```python
from build123d import *

# Parameters (mm, degrees)
EXTRUDE_1_DEPTH      = 1.5
CUT_EXTRUDE_1_DEPTH  = 1.5
SKETCH_3_R           = 2
CUT_EXTRUDE_2_DEPTH  = 1.5
SKETCH_4_W           = 80
SKETCH_4_H           = 5
EXTRUDE_2_DEPTH      = 1.5
FILLET_1_R           = 2
SKETCH_5_OUTSIDE_W   = 163.618
SKETCH_5_OUTSIDE_H   = 213.618
SKETCH_5_OUTSIDE_W_2 = 80
SKETCH_5_OUTSIDE_H_2 = 170
CUT_EXTRUDE_3_DEPTH  = 193.943644622
SKETCH_6_R           = 1.5
CUT_EXTRUDE_4_DEPTH  = 184.377343202


with BuildPart() as part:
    # 草图1 → 凸台-拉伸1 (new body)
    with BuildSketch(Plane.XY):
        Polygon((80, 90), (100, 90), (100, 70), (80, 70), (80, 0), (0, 0), (0, 70), (-20, 70), (-20, 90), (0, 90), (0, 160), (80, 160), align=None)
    extrude(amount=EXTRUDE_1_DEPTH)

    # 草图2 → 切除-拉伸1 (cut)
    with BuildSketch(Plane.XY.offset(1.5)):
        with BuildLine():
            Line((57.5, 152.25), (80, 152.25))
            Line((80, 152.25), (80, 157.75))
            Line((80, 157.75), (57.5, 157.75))
            ThreePointArc((57.5, 157.75), (54.75, 155), (57.5, 152.25))
        make_face()
        with BuildLine():
            Line((22.5, 152.25), (0, 152.25))
            Line((0, 152.25), (0, 157.75))
            Line((0, 157.75), (22.5, 157.75))
            ThreePointArc((22.5, 157.75), (25.25, 155), (22.5, 152.25))
        make_face()
        with BuildLine():
            Line((57.5, 102.25), (80, 102.25))
            Line((80, 102.25), (80, 107.75))
            Line((80, 107.75), (57.5, 107.75))
            ThreePointArc((57.5, 107.75), (54.75, 105), (57.5, 102.25))
        make_face()
        with BuildLine():
            Line((22.5, 107.75), (0, 107.75))
            Line((0, 107.75), (0, 102.25))
            Line((0, 102.25), (22.5, 102.25))
            ThreePointArc((22.5, 102.25), (25.25, 105), (22.5, 107.75))
        make_face()
        with BuildLine():
            Line((22.5, 57.75), (0, 57.75))
            Line((0, 57.75), (0, 52.25))
            Line((0, 52.25), (22.5, 52.25))
            ThreePointArc((22.5, 52.25), (25.25, 55), (22.5, 57.75))
        make_face()
        with BuildLine():
            Line((57.5, 52.25), (80, 52.25))
            Line((80, 52.25), (80, 57.75))
            Line((80, 57.75), (57.5, 57.75))
            ThreePointArc((57.5, 57.75), (54.75, 55), (57.5, 52.25))
        make_face()
        with BuildLine():
            Line((22.5, 7.75), (0, 7.75))
            Line((0, 7.75), (0, 2.25))
            Line((0, 2.25), (22.5, 2.25))
            ThreePointArc((22.5, 2.25), (25.25, 5), (22.5, 7.75))
        make_face()
        with BuildLine():
            Line((57.5, 7.75), (80, 7.75))
            Line((80, 7.75), (80, 2.25))
            Line((80, 2.25), (57.5, 2.25))
            ThreePointArc((57.5, 2.25), (54.75, 5), (57.5, 7.75))
        make_face()
    extrude(amount=-CUT_EXTRUDE_1_DEPTH, mode=Mode.SUBTRACT)

    # 草图3 → 切除-拉伸2 (cut)
    with BuildSketch(Plane.XY.offset(1.5)):
        with Locations((90, 80)):
            Circle(SKETCH_3_R)
        with Locations((-10, 80)):
            Circle(SKETCH_3_R)
    extrude(amount=-CUT_EXTRUDE_2_DEPTH, mode=Mode.SUBTRACT)

    # 草图4 → 凸台-拉伸2 (add)
    with BuildSketch(Plane(origin=(0, 0, 0), x_dir=(-1, 0, 0), z_dir=(0, 0, -1))):
        with Locations((-40, 162.5)):
            Rectangle(SKETCH_4_W, SKETCH_4_H)
        with Locations((-40, -2.5)):
            Rectangle(SKETCH_4_W, SKETCH_4_H)
    extrude(amount=-EXTRUDE_2_DEPTH)

    # 圆角1
    fillet_1_edges = [part.edges().sort_by_distance(p)[0] for p in [
        (0, 165, 0.75),
        (80, 165, 0.75),
        (0, -5, 0.75),
        (80, -5, 0.75),
    ]]
    fillet(fillet_1_edges, radius=FILLET_1_R)

    # 草图5 outside → 切除-拉伸3 (cut, through all)
    with BuildSketch(Plane.XY.offset(1.5)):
        with Locations((40, 80)):
            Rectangle(SKETCH_5_OUTSIDE_W, SKETCH_5_OUTSIDE_H)
        with Locations((40, 80)):
            Rectangle(SKETCH_5_OUTSIDE_W_2, SKETCH_5_OUTSIDE_H_2, mode=Mode.SUBTRACT)
    extrude(amount=-CUT_EXTRUDE_3_DEPTH, mode=Mode.SUBTRACT)

    # 草图6 → 切除-拉伸4 (cut, through all)
    with BuildSketch(Plane(origin=(0, 0, 0), x_dir=(-1, 0, 0), z_dir=(0, 0, -1))):
        with Locations((-35, 85)):
            Circle(SKETCH_6_R)
        with Locations((-35, 75)):
            Circle(SKETCH_6_R)
        with Locations(Location((-45, 75, 0), (0, 0, 180))):
            Circle(SKETCH_6_R)
        with Locations(Location((-45, 85, 0), (0, 0, 180))):
            Circle(SKETCH_6_R)
    extrude(amount=-CUT_EXTRUDE_4_DEPTH, mode=Mode.SUBTRACT)


solid = part.part
```
For this review, take the finished solid that the model builds, in its own axes (mm). Coordinates: 2 decimals unless noted, no trailing zeros. Loops run counter-clockwise (first coordinate to the right, second up) from the corner with the lowest first, then second, coordinate; pieces in that order, holes last. Notation, with made-up numbers: (-38, -35) -> (7, -35) arc R14 cw to (7, -29) -> close; hole circle Ø8 at (-35.75, 5). An arc over 180 degrees is marked (long way). Return JSON: item names as keys, results as strings. Group by question number.
(1) Mouldability with a two-part tool opening along Y and no side actions: class faces 1 (the flat face through (41, 81, 0)), 2 (the cylindrical face through (43.89, 73.99, 0.74)), 3 (the cylindrical face through (35.195, 86.487, 0.74)) as pulls with the +Y half, pulls with the -Y half, needs draft (parallel to the pull), parting line crosses it, or undercut.
(2) Consider section A-A, the plane x = 62.5. Give the boundary of the cut face in (y, z).
(3) For pin 1 Ø3 at (x, y) = (28, 32.5) entering from -Z, flat-tipped, find the tip position at first contact; note if it passes through.
(4) Consider section C-C, the plane y = 105. Give the boundary of the cut face in (x, z).
(5) Consider section B-B, the plane z = 0.4. Count the separate pieces of the cut face and the enclosed holes in it, plus the area to 3 significant figures.
(6) To check wall thickness, follow L1, parallel to Y at x = 13.5, z = 0.95; L2, parallel to X at y = 75, z = 0.4; L3, parallel to Y at x = 35, z = 0.5. State the ranges of each line that lie inside material, in increasing order.
Results below:
{
 "1": {"face 1": "needs draft", "face 2": "undercut", "face 3": "undercut"},
 "2": {"outline": "(-5, 0) -> (2.25, 0) -> (2.25, 1.5) -> (-5, 1.5) -> close; (7.75, 0) -> (52.25, 0) -> (52.25, 1.5) -> (7.75, 1.5) -> close; (57.75, 0) -> (102.25, 0) -> (102.25, 1.5) -> (57.75, 1.5) -> close; (107.75, 0) -> (152.25, 0) -> (152.25, 1.5) -> (107.75, 1.5) -> close; (157.75, 0) -> (165, 0) -> (165, 1.5) -> (157.75, 1.5) -> close"},
 "3": {"pin 1": "stops at z = 0"},
 "4": {"outline": "(25.25, 0) -> (54.75, 0) -> (54.75, 1.5) -> (25.25, 1.5) -> close"},
 "5": {"separate pieces": "1", "enclosed holes": "4", "area": "12,500 mm2"},
 "6": {"L1": "y = -5 to 2.25, 7.75 to 52.25, 57.75 to 102.25, 107.75 to 152.25, 157.75 to 165", "L2": "x = 0 to 33.5, 36.5 to 43.5, 46.5 to 80", "L3": "y = -5 to 73.5, 76.5 to 83.5, 86.5 to 165"}
}
